Autodesk Inventor part; units mm, degrees
ref_plane "YZ Plane" through (0, 0, 0) normal (1, 0, 0) x (0, 1, 0)
ref_plane "XZ Plane" through (0, 0, 0) normal (0, 1, 0) x (-1, 0, 0)
ref_plane "XY Plane" through (0, 0, 0) normal (0, 0, 1) x (1, 0, 0)
sketch "Sketch1" plane through (0, 0, 0) normal (0, 1, 0) x (-1, 0, 0)
  line L0 (33.8585, -6) -> (-33.8585, -6)
  line L1 (-34.295, -2.5) -> (34.295, -2.5)
  line L2 (0.5017, -38.45) -> (-0.4983, -38.45)
  line L3 (-0.4983, -38.45) -> (-0.4983, -38.85)
  line L4 (-0.4983, -38.85) -> (0.5017, -38.85)
  line L5 (0.5017, -38.85) -> (0.5017, -38.45)
  line L6 (0.5017, -38.45) -> (-0.4983, -38.85) construction
  line L7 (-0.4983, -38.45) -> (0.5017, -38.85) construction
  line L8 (9.6888, -37.2126) -> (8.7179, -37.452)
  line L9 (8.7179, -37.452) -> (8.8136, -37.8403)
  line L10 (8.8136, -37.8403) -> (9.7846, -37.601)
  line L11 (9.7846, -37.601) -> (9.6888, -37.2126)
  line L12 (18.3129, -33.8126) -> (17.4274, -34.2773)
  line L13 (17.4274, -34.2773) -> (17.6133, -34.6315)
  line L14 (17.6133, -34.6315) -> (18.4987, -34.1668)
  line L15 (18.4987, -34.1668) -> (18.3129, -33.8126)
  line L16 (25.8726, -28.4475) -> (25.1241, -29.1107)
  line L17 (25.1241, -29.1107) -> (25.3893, -29.4101)
  line L18 (25.3893, -29.4101) -> (26.1379, -28.7469)
  line L19 (26.1379, -28.7469) -> (25.8726, -28.4475)
  line L20 (31.9287, -21.4292) -> (31.3607, -22.2522)
  line L21 (31.3607, -22.2522) -> (31.6899, -22.4794)
  line L22 (31.6899, -22.4794) -> (32.2579, -21.6564)
  line L23 (32.2579, -21.6564) -> (31.9287, -21.4292)
  line L24 (36.1293, -13.1654) -> (35.7747, -14.1005)
  line L25 (35.7747, -14.1005) -> (36.1487, -14.2423)
  line L26 (36.1487, -14.2423) -> (36.5033, -13.3073)
  line L27 (36.5033, -13.3073) -> (36.1293, -13.1654)
  line L28 (38.2301, -4.1366) -> (38.1096, -5.1293)
  line L29 (38.1096, -5.1293) -> (38.5067, -5.1775)
  line L30 (38.5067, -5.1775) -> (38.6272, -4.1848)
  line L31 (38.6272, -4.1848) -> (38.2301, -4.1366)
  line L32 (38.1092, 5.1327) -> (38.2297, 4.14)
  line L33 (38.2297, 4.14) -> (38.6268, 4.1882)
  line L34 (38.6268, 4.1882) -> (38.5063, 5.1809)
  line L35 (38.5063, 5.1809) -> (38.1092, 5.1327)
  line L36 (35.7735, 14.1037) -> (36.1281, 13.1687)
  line L37 (36.1281, 13.1687) -> (36.5021, 13.3105)
  line L38 (36.5021, 13.3105) -> (36.1475, 14.2455)
  line L39 (36.1475, 14.2455) -> (35.7735, 14.1037)
  line L40 (31.3587, 22.255) -> (31.9268, 21.432)
  line L41 (31.9268, 21.432) -> (32.256, 21.6592)
  line L42 (32.256, 21.6592) -> (31.6879, 22.4822)
  line L43 (31.6879, 22.4822) -> (31.3587, 22.255)
  line L44 (25.1215, 29.1129) -> (25.87, 28.4498)
  line L45 (25.87, 28.4498) -> (26.1353, 28.7492)
  line L46 (26.1353, 28.7492) -> (25.3868, 29.4123)
  line L47 (25.3868, 29.4123) -> (25.1215, 29.1129)
  line L48 (17.4244, 34.2789) -> (18.3098, 33.8142)
  line L49 (18.3098, 33.8142) -> (18.4957, 34.1684)
  line L50 (18.4957, 34.1684) -> (17.6102, 34.6331)
  line L51 (17.6102, 34.6331) -> (17.4244, 34.2789)
  line L52 (8.7145, 37.4528) -> (9.6855, 37.2135)
  line L53 (9.6855, 37.2135) -> (9.7812, 37.6018)
  line L54 (9.7812, 37.6018) -> (8.8103, 37.8412)
  line L55 (8.8103, 37.8412) -> (8.7145, 37.4528)
  line L56 (-0.5017, 38.45) -> (0.4983, 38.45)
  line L57 (0.4983, 38.45) -> (0.4983, 38.85)
  line L58 (0.4983, 38.85) -> (-0.5017, 38.85)
  line L59 (-0.5017, 38.85) -> (-0.5017, 38.45)
  line L60 (-9.6888, 37.2126) -> (-8.7179, 37.452)
  line L61 (-8.7179, 37.452) -> (-8.8136, 37.8403)
  line L62 (-8.8136, 37.8403) -> (-9.7846, 37.601)
  line L63 (-9.7846, 37.601) -> (-9.6888, 37.2126)
  line L64 (-18.3129, 33.8126) -> (-17.4274, 34.2773)
  line L65 (-17.4274, 34.2773) -> (-17.6133, 34.6315)
  line L66 (-17.6133, 34.6315) -> (-18.4987, 34.1668)
  line L67 (-18.4987, 34.1668) -> (-18.3129, 33.8126)
  line L68 (-25.8726, 28.4475) -> (-25.1241, 29.1107)
  line L69 (-25.1241, 29.1107) -> (-25.3893, 29.4101)
  line L70 (-25.3893, 29.4101) -> (-26.1379, 28.7469)
  line L71 (-26.1379, 28.7469) -> (-25.8726, 28.4475)
  line L72 (-31.9287, 21.4292) -> (-31.3607, 22.2522)
  line L73 (-31.3607, 22.2522) -> (-31.6899, 22.4794)
  line L74 (-31.6899, 22.4794) -> (-32.2579, 21.6564)
  line L75 (-32.2579, 21.6564) -> (-31.9287, 21.4292)
  line L76 (-36.1293, 13.1654) -> (-35.7747, 14.1005)
  line L77 (-35.7747, 14.1005) -> (-36.1487, 14.2423)
  line L78 (-36.1487, 14.2423) -> (-36.5033, 13.3073)
  line L79 (-36.5033, 13.3073) -> (-36.1293, 13.1654)
  line L80 (-38.2301, 4.1366) -> (-38.1096, 5.1293)
  line L81 (-38.1096, 5.1293) -> (-38.5067, 5.1775)
  line L82 (-38.5067, 5.1775) -> (-38.6272, 4.1848)
  line L83 (-38.6272, 4.1848) -> (-38.2301, 4.1366)
  line L84 (-38.1092, -5.1327) -> (-38.2297, -4.14)
  line L85 (-38.2297, -4.14) -> (-38.6268, -4.1882)
  line L86 (-38.6268, -4.1882) -> (-38.5063, -5.1809)
  line L87 (-38.5063, -5.1809) -> (-38.1092, -5.1327)
  line L88 (-35.7735, -14.1037) -> (-36.1281, -13.1687)
  line L89 (-36.1281, -13.1687) -> (-36.5021, -13.3105)
  line L90 (-36.5021, -13.3105) -> (-36.1475, -14.2455)
  line L91 (-36.1475, -14.2455) -> (-35.7735, -14.1037)
  line L92 (-31.3587, -22.255) -> (-31.9268, -21.432)
  line L93 (-31.9268, -21.432) -> (-32.256, -21.6592)
  line L94 (-32.256, -21.6592) -> (-31.6879, -22.4822)
  line L95 (-31.6879, -22.4822) -> (-31.3587, -22.255)
  line L96 (-25.1215, -29.1129) -> (-25.87, -28.4498)
  line L97 (-25.87, -28.4498) -> (-26.1353, -28.7492)
  line L98 (-26.1353, -28.7492) -> (-25.3868, -29.4123)
  line L99 (-25.3868, -29.4123) -> (-25.1215, -29.1129)
  line L100 (-17.4244, -34.2789) -> (-18.3098, -33.8142)
  line L101 (-18.3098, -33.8142) -> (-18.4957, -34.1684)
  line L102 (-18.4957, -34.1684) -> (-17.6102, -34.6331)
  line L103 (-17.6102, -34.6331) -> (-17.4244, -34.2789)
  line L104 (-8.7145, -37.4528) -> (-9.6855, -37.2135)
  line L105 (-9.6855, -37.2135) -> (-9.7812, -37.6018)
  line L106 (-9.7812, -37.6018) -> (-8.8103, -37.8412)
  line L107 (-8.8103, -37.8412) -> (-8.7145, -37.4528)
  arc A0 (-33.6574, 19) -> (32.0907, -21.5409) centre (0, 0) ccw
  arc A1 (33.6574, -19) -> (33.6574, 19) centre (0, 0) ccw
  arc A2 (32.0887, 21.5438) -> (-32.0907, 21.5409) centre (0, 0) ccw
  line L108 (36.1642, -3.8857) -> (36.1642, -3.8892)
  line L109 (36.1642, -4.8931) -> (36.1642, -4.8965)
  line L110 (-34.9312, -4.7468) -> (-34.9312, -4.7433)
  line L111 (-34.9312, -3.7395) -> (-34.9312, -3.736)
  line L112 (33.6574, -19) -> (28.66, -19)
  line L113 (-28.66, -19) -> (-33.6574, -19)
  line L114 (-33.6574, 19) -> (-28.66, 19)
  line L115 (28.66, 19) -> (33.6574, 19)
  arc A3 (28.66, -19) -> (33.8585, -6) centre (0, 0) ccw
  arc A4 (34.295, -2.5) -> (28.66, 19) centre (0, 0) ccw
  arc A5 (-28.66, 19) -> (-34.295, -2.5) centre (0, 0) ccw
  arc A6 (-33.8585, -6) -> (-28.66, -19) centre (0, 0) ccw
  point P0 (0.0017, -38.65)
  point P1 (35.9587, -14.1702)
  point P2 (36.3132, -13.2352)
  point P3 (38.3049, -5.153)
  point P4 (38.4254, -4.1603)
  point P5 (38.4251, 4.1637)
  point P6 (38.3045, 5.1564)
  point P7 (36.3121, 13.2384)
  point P8 (35.9574, 14.1734)
  point P9 (-35.9587, 14.1702)
  point P10 (-36.3132, 13.2352)
  point P11 (-38.3049, 5.153)
  point P12 (-38.4254, 4.1603)
  point P13 (-38.4251, -4.1637)
  point P14 (-38.3045, -5.1564)
  point P15 (-36.3121, -13.2384)
  point P16 (-35.9574, -14.1734)
  dimension "d2" = 2.5
  dimension "d3" = 3.5
  dimension "d10" = 1
  dimension "d11" = 0.4
  dimension "d14" = 360
  dimension "d18" = 38.65
  dimension "d19" = 4.9974
extrude "Extrusion1" add sketch "Sketch1" along normal blind 11.5 contours L0 A6 L113 A0 L91 L88 L89 L87 L84 L85 L83 L80 L81 L79 L76 L77 L114 A5 L1 A4 L115 A1 L39 L36 L37 L35 L32 L33 L31 L28 L29 L27 L24 L25 L112 A3 | A1 L27 L26 L25 | L25 L24 L27 A1 | A0 L89 L88 L91 | L91 L90 L89 A0 | A1 L31 L30 L29 | L29 L28 L31 A1 | A0 L85 L84 L87 | L87 L86 L85 A0 | A1 L35 L34 L33 | L33 L32 L35 A1 | A0 L81 L80 L83 | L83 L82 L81 A0 | A1 L39 L38 L37 | L37 L36 L39 A1 | A0 L77 L76 L79 | L79 L78 L77 A0
sketch "Sketch2" plane through (0, 11.5, 0) normal (0, 1, 0) x (1, 0, 0)
  arc A0 (33.8585, 6) -> (28.66, 19) centre (0, 0) ccw
  line L0 (34.295, 2.5) -> (-34.295, 2.5)
  line L1 (-3.804, 9) -> (7.0469, 9)
  line L2 (33.1873, 9) -> (-33.1873, 9)
  line L3 (-28.66, 19) -> (-33.6574, 19)
  line L4 (-33.6574, -19) -> (-28.66, -19)
  line L5 (-28.66, -19) -> (-36.8951, -19)
  arc A1 (-34.295, 2.5) -> (-28.66, -19) centre (0, 0) ccw
  arc A2 (28.66, -19) -> (34.295, 2.5) centre (0, 0) ccw
  arc A3 (36.8951, -19) -> (36.8951, 19) centre (0, 0) ccw
  arc A4 (-36.8951, 19) -> (-36.8951, -19) centre (0, 0) ccw
  arc A5 (33.1873, 9) -> (28.66, 19) centre (0, 0) ccw
  arc A6 (-28.66, 19) -> (-33.1873, 9) centre (0, 0) ccw
  line L6 (36.8951, 19) -> (28.66, 19)
  line L7 (-28.66, 19) -> (-36.8951, 19)
  line L8 (-31.7819, -19) -> (-28.66, -19)
  line L9 (28.66, -19) -> (36.8951, -19)
  line L10 (-30.5962, 19) -> (-28.66, 19)
  line L11 (28.66, 19) -> (36.8951, 19)
  point P0 (28.66, 19)
  point P1 (7.0469, 9)
  dimension "d24" = 41.5
  dimension "d25" = 6.5
extrude "Extrusion2" add sketch "Sketch2" along normal blind 2
sketch "Sketch3" plane through (-34.295, 0, -2.5) normal (0, 0, 1) x (1, 0, 0)
  line L0 (0, 13.5) -> (68.59, 13.5)
  line L1 (0, 0) -> (0, 13.5)
  point P0 (34.295, 0)
  point P1 (34.0614, 4.8894)
  dimension "d28" = 8.6106
  dimension "d29" = 34.0614
hole "Hole1" at (-0.2336, 4.8894, -2.5) direction (0, 0, -1) diameter 2.6416 depth 10.979
properties part number "AQS_Mount_3DPrint"
Input: part model. Units: mm. Frame: model coordinates. A direction names the side the tool comes from. Round coordinates to 2 decimals unless told otherwise and drop trailing zeros. Write each loop counter-clockwise with the first axis right and the second up, starting at its lowest first coordinate (ties: lowest second). Pieces come first, ordered by that corner, then holes. Notation, with made-up numbers: (78, -16.5) - (137, -16.5) arc R14 cw to (137, 1.5) - close; hole circle Ø7 at (-30, 72.5). An arc over 180 degrees is marked (long way). Write item = value, one per line.
(1) Section query C-C on y = 12.5. Output: boundary loops of the cut face in (x, z) (3 decimals).
Geometry check:
outline = (-36.895, -19) - (-28.66, -19) arc R34.387 cw to (-33.187, -9) - (33.187, -9) arc R34.385 cw to (28.66, -19) - (36.895, -19) arc R41.5 ccw to (36.895, 19) - (28.66, 19) arc R34.386 cw to (34.295, -2.5) - (-34.295, -2.5) arc R34.386 cw to (-28.66, 19) - (-36.895, 19) arc R41.5 ccw to start
(2) Section query D-D on x = 7. Output: boundary loops of the cut face in (y, z), then the cut area to 4 significant figures.
Geometry check:
outline = (0, -6) - (11.5, -6) - (11.5, -9) - (13.5, -9) - (13.5, -2.5) - (0, -2.5) - close
area = 53.25 mm^2
(3) Section query A-A on z = -15. Output: boundary loops of the cut face in (x, y).
Geometry check:
outline = (-38.69, 11.5) - (-35.62, 11.5) - (-35.62, 0) - (-30.94, 0) - (-30.94, 13.5) - (-38.69, 13.5) - close; (30.94, 0) - (35.62, 0) - (35.62, 11.5) - (38.69, 11.5) - (38.69, 13.5) - (30.94, 13.5) - close
(4) Contact query for flat-ended pins moving along their axis: pin 1 Ø3 at (y, z) = (11, -9) entering from -X; pin 2 Ø0.6 at (x, y) = (7.5, 13) entering from -Z; pin 3 Ø6 at (y, z) = (3, 1.5) entering from -X. Output: stop coordinate, or through.
Geometry check:
pin_1 = -40.8
pin_2 = -9
pin_3 = -38.65
(5) Section query B-B on x = -31. Output: boundary loops of the cut face in (y, z), then the cut area to 3 significant figures.
Geometry check:
outline = (0, -19) - (13.5, -19) - (13.5, -14.88) - (0, -14.88) - close; (0, -6) - (11.5, -6) - (11.5, -9) - (13.5, -9) - (13.5, -2.5) - (0, -2.5) - close; (0, 14.88) - (13.5, 14.88) - (13.5, 19) - (0, 19) - close
area = 165 mm^2
(6) Material intervals for probe 1 along Z at (x, y) = (-12, 4.25); probe 2 along Z at (x, y) = (-12, 13); probe 3 along Y at (x, z) = (28, -7.5), sorted ascending.
Geometry check:
probe_1 = -6 to -2.5
probe_2 = -9 to -2.5
probe_3 = 11.5 to 13.5
(7) Pull-direction query (X, two-part tool) for faces 1 (the flat face through (0, 7, -2.5)), 2 (the cylindrical face through (-38.65, 5.67, 0.06)), 3 (the flat face through (3, 0, -3)); classes: +X half, -X half, draft (parallel to the pull), parting line (faces both ways), or undercut.
Geometry check:
face_1 = undercut
face_2 = -X half
face_3 = draft
(8) Access query for faces 4 (the flat face through (0, 7, -6)), 5 (the flat face through (39, 11.5, 0)), 6 (the flat face through (-39, 11.5, 0)). Directions: +Z, -Z, +X, -X, +Y, -Y. A direction counts if a zero-diameter tool reaches every point of the face in a straight line with its end or side. Return the directions, or none.
Geometry check:
face_4 = -Y
face_5 = +X, -Y
face_6 = -X, -Y
